Autodesk Inventor part; units mm, degrees
ref_plane "Work Plane1" through (8.5, -35.5, -35.5) normal (0, 0, -1) x (-1, 0, 0)
ref_plane "YZ Plane" through (0, 0, 0) normal (1, 0, 0) x (0, 1, 0)
ref_plane "XZ Plane" through (0, 0, 0) normal (0, 1, 0) x (-1, 0, 0)
ref_plane "Work Plane1" through (8.5, -35.5, -35.5) normal (0, 0, -1) x (-1, 0, 0)
sketch "Sketch1" plane through (8.5, -35.5, -35.5) normal (0, 0, -1) x (-1, 0, 0)
  circle A0 centre (0, 0) radius 3
  circle A1 centre (0, 0) radius 6
  circle A2 centre (-36.75, -21.2176) radius 3
  circle A3 centre (-36.75, -21.2176) radius 6
  circle A4 centre (-36.75, 21.2176) radius 6
  circle A5 centre (-36.75, 21.2176) radius 3
  line L0 (-36.75, -46.2176) -> (28, -46.2176)
  line L1 (28, -46.2176) -> (28, 0)
  line L2 (-36.75, -46.2176) -> (-59, -46.2176)
  line L3 (-59, -46.2176) -> (-59, 34.5)
  line L4 (-59, 34.5) -> (28, 34.5)
  line L5 (34.5, 35.5) -> (-17.5, 35.5)
  line L6 (28, 34.5) -> (28, 0)
  circle A6 centre (-24.5, 0) radius 11
  circle A7 centre (-24.5, 0) radius 15
  point P0 (8.5, 35.5)
  dimension "d3" = 30
extrude "Extrusion1" add sketch "Sketch1" along normal blind 5 contours A1 | A3 | A4 | L2 L3 L4 L6 L1 L0
sketch "Sketch2" plane through (-19.5, -81.7176, -35.5) normal (-1, 0, 0) x (0, 0, 1)
  line L0 (0, 0) -> (0, 80.7176)
  line L1 (0, 80.7176) -> (-5, 80.7176)
  line L2 (-5, 0) -> (-5, 80.7176)
  line L3 (0, 0) -> (-5, 0)
  point P0 (35.5, 81.7176)
extrude "Extrusion2" add sketch "Sketch2" along normal blind 5
sketch "Sketch3" plane through (67.5, -81.7176, -40.5) normal (0, -1, 0) x (1, 0, 0)
  line L0 (0, 5) -> (-92, 5)
  line L1 (-92, 0) -> (-92, 5)
  line L2 (0, 0) -> (-92, 0)
  line L3 (0, 5) -> (0, 0)
  point P0 (-67.5, 40.5)
extrude "Extrusion3" add sketch "Sketch3" along normal blind 5
sketch "Sketch4" plane through (8.5, -35.5, -35.5) normal (0, 0, 1) x (1, 0, 0)
  line L0 (-28, -46.2176) -> (-28, 34.5)
  line L1 (-28, -46.2176) -> (59, -46.2176)
  line L2 (59, -51.2176) -> (-33, -51.2176)
  line L3 (-33, 34.5) -> (-33, -51.2176)
  line L4 (59, 34.5) -> (59, -51.2176)
  line L5 (59, 34.5) -> (-33, 34.5)
  line L6 (-28, -46.2176) -> (-33, -46.2176)
  line L7 (-33, 34.5) -> (-33, -51.2176)
extrude "Extrusion4" add sketch "Sketch4" along normal blind 75 contours L1 L4 L2 L3 L6
sketch "Sketch5" plane through (67.5, -86.7176, -40.5) normal (0, -1, 0) x (1, 0, 0)
  line L0 (-92, 5) -> (-92, 80)
  line L1 (-92, 80) -> (-77.75, 80)
  line L2 (-92, 80) -> (0, 80)
  line L3 (-77.75, 80) -> (-37.75, 80)
  line L4 (-37.75, 80) -> (-37.75, 65)
  line L5 (-37.75, 65) -> (-77.75, 65)
  circle A0 centre (-77.75, 65) radius 4.25
  circle A1 centre (-37.75, 65) radius 4.25
  point P0 (-67.5, 40.5)
  dimension "d14" = 14.25
  dimension "d15" = 40
  dimension "d16" = 15
  dimension "d17" = 8.5
  dimension "d18" = 8.5
extrude "Extrusion5" cut sketch "Sketch5" against normal through all
sketch "Sketch6" plane through (67.5, -1, -35.5) normal (0, 1, 0) x (1, 0, 0)
  line L0 (0, 0) -> (-92, 0)
  line L1 (0, 0) -> (0, 5)
  line L2 (0, 5) -> (-92, 5)
  line L3 (-92, 0) -> (-92, 5)
  point P0 (-67.5, -35.5)
extrude "Extrusion6" add sketch "Sketch6" along normal blind 20
sketch "Sketch7" plane through (67.5, 19, -35.5) normal (0, 1, 0) x (1, 0, 0)
  circle A0 centre (-67.5, -35.5) radius 31
  circle A1 centre (-67.5, -35.5) radius 31
  circle A2 centre (-67.5, -35.5) radius 31
  line L0 (-67.5, -66.5) -> (-67.5, -75)
  line L1 (0, -75) -> (-92, -75)
  line L2 (0, 5) -> (0, -75)
  line L3 (-67.5, -75) -> (0, -75)
  line L4 (0, -75) -> (0, 5)
  line L5 (-65, -20.5) -> (-65, 0)
  line L6 (-65, -4.601) -> (-65, 0)
  line L7 (-92, 5) -> (-92, 0)
  line L8 (-92, 0) -> (0, 0)
  line L9 (0, 0) -> (0, 5)
  line L10 (0, 5) -> (-92, 5)
  point P0 (-65, -4.601)
extrude "Extrusion7" add sketch "Sketch7" along normal blind 20 contours A0 L5 L8 L2 L1 L0 | L8 L7 L10 L2
sketch "Sketch10" plane through (8.5, -35.5, 39.5) normal (0, 0, 1) x (1, 0, 0)
  line L0 (59, -51.2176) -> (59, -46.2176)
  line L1 (59, -46.2176) -> (-33, -46.2176)
  line L2 (-33, -46.2176) -> (-33, -51.2176)
  line L3 (-33, -51.2176) -> (59, -51.2176)
  point P0 (-8.5, 35.5)
extrude "Extrusion10" cut sketch "Sketch10" against normal up to surface (75 mm away)
sketch "Sketch11" plane through (0, 19, 39.5) normal (0, 0, 1) x (1, 0, 0)
  line L0 (0, 0) -> (67.5, 0)
  line L1 (67.5, 0) -> (67.5, 20)
  line L2 (0, 20) -> (67.5, 20)
  line L3 (0, 0) -> (0, 20)
  point P0 (0, -19)
extrude "Extrusion11" add sketch "Sketch11" along normal blind 10
sketch "Sketch12" plane through (67.5, 19, -35.5) normal (0, -1, 0) x (1, 0, 0)
  line L0 (-67.5, 66.5) -> (-67.5, 85)
  line L1 (-67.5, 85) -> (0, 85)
  line L2 (-67.5, 85) -> (0, 85)
  line L3 (0, 85) -> (0, 75)
  line L4 (0, 0) -> (0, 85)
  line L5 (0, 75) -> (-67.5, 75)
  line L6 (-67.5, 75) -> (-67.5, 85)
  point P0 (-67.5, 35.5)
  dimension "d35" = 10
extrude "Extrusion12" add sketch "Sketch12" along normal blind 20
sketch "Sketch13" plane through (0, 19, 49.5) normal (0, 0, 1) x (1, 0, 0)
  line L0 (67.5, 20) -> (67.5, -20)
  line L1 (67.5, 20) -> (0, 20)
  line L2 (0, 20) -> (0, -20)
  line L3 (67.5, -20) -> (0, -20)
  point P0 (0, -19)
extrude "Extrusion13" add sketch "Sketch13" along normal blind 59.488
sketch "Sketch14" plane through (67.5, -1, -35.5) normal (0, -1, 0) x (1, 0, 0)
  line L0 (-53.25, 129.488) -> (-13.25, 129.488)
  circle A0 centre (-53.25, 129.488) radius 4.25
  circle A1 centre (-13.25, 129.488) radius 4.25
  point P0 (-67.5, 35.5)
  point P1 (-67.5, 144.488)
  dimension "d43" = 40
  dimension "d44" = 8.5
  dimension "d45" = 8.5
extrude "Extrusion14" cut sketch "Sketch14" against normal up to surface (40 mm away)
sketch "Sketch15" plane through (67.5, -86.7176, -40.5) normal (1, 0, 0) x (0, 0, -1)
  line L0 (-5, 105.7176) -> (-5, 0)
  line L1 (0, 0) -> (-5, 0)
  line L2 (0, 0) -> (0, 125.7176)
  line L3 (0, 125.7176) -> (-149.488, 125.7176)
  line L4 (-149.488, 85.7176) -> (-149.488, 125.7176)
  line L5 (-80, 85.7176) -> (-149.488, 85.7176)
  line L6 (-80, 105.7176) -> (-80, 85.7176)
  line L7 (-5, 105.7176) -> (-80, 105.7176)
  point P0 (-40.5, 86.7176)
extrude "Extrusion15" add sketch "Sketch15" along normal blind 1
sketch "Sketch16" plane through (0, 19, 31) normal (-1, 0, 0) x (0, 0, 1)
  line L0 (77.988, 20) -> (77.988, -20)
  line L1 (77.988, 0) -> (42.988, 0)
  circle A0 centre (42.988, 0) radius 4.25
  point P0 (-31, -19)
  dimension "d50" = 35
  dimension "d51" = 8.5
extrude "Extrusion16" cut sketch "Sketch16" against normal up to surface (68.5 mm away)
sketch "Sketch17" plane through (67.5, 39, -35.5) normal (0, 1, 0) x (1, 0, 0)
  circle A0 centre (-53.25, -129.488) radius 4.25
  line L0 (-53.25, -129.488) -> (-33.25, -129.488)
  line L1 (-33.25, -129.488) -> (-33.25, -99.488)
  circle A1 centre (-33.25, -99.488) radius 4.25
  point P0 (-67.5, -35.5)
  dimension "d54" = 20
  dimension "d55" = 30
  dimension "d56" = 8.5
extrude "Extrusion17" cut sketch "Sketch17" against normal up to surface (40 mm away) contours A1
sketch "Sketch18" plane through (8.5, -35.5, -35.5) normal (0, 0, 1) x (1, 0, 0)
  line L0 (-6, 54.5) -> (60, 54.5)
  line L1 (-6, 54.5) -> (-6, 74.5)
  line L2 (-33, 74.5) -> (-6, 74.5)
  line L3 (-33, 74.5) -> (-33, -51.2176)
  line L4 (-33, -51.2176) -> (60, -51.2176)
  line L5 (60, 54.5) -> (60, -51.2176)
  circle A0 centre (0, 0) radius 3
  circle A1 centre (36.75, -21.2176) radius 3
  circle A2 centre (36.75, 21.2176) radius 3
  circle A3 centre (24.5, 0) radius 15
  circle A4 centre (36.75, 21.2176) radius 6.5
  circle A5 centre (36.75, -21.2176) radius 6.5
  circle A6 centre (0, 0) radius 3
  circle A7 centre (0, 0) radius 6.5
  point P0 (-8.5, 35.5)
  dimension "d59" = 13
  dimension "d60" = 13
  dimension "d61" = 13
extrude "Extrusion18" add sketch "Sketch18" along normal up to surface (4.601 mm away) contours L0 L5 L4 L3 L2 L1
properties part number "motor_connector_left"
CAD build for the part. Positions are in the model's coordinates, mm. A direction names the side the tool comes from. Give positions to 0.01 mm unless a question says otherwise; leave off trailing zeros. Write each loop counter-clockwise with the first axis right and the second up, starting at its lowest first coordinate (ties: lowest second). Pieces come first, ordered by that corner, then holes. Notation, with made-up numbers: M 51.5,66.25 L 61.5,66.25 A9 cw 61.5,81.25 Z; hole C -8,52 d10. An arc over 180 degrees is marked long. Return JSON: item names as keys, results as strings. Group by question number.
(1) Band-saw the part on B-B (x = 20.5). Give the cut face in (y, z), and give its area (3 significant figures).
(2) Band-saw the part on D-D (y = -5). Give the cut face in (x, z), and give its area (3 significant figures).
(3) Band-saw the part on A-A (x = 54.25). Give the cut face in (y, z).
(4) Flat gauge pins, fed straight in: pin 1 Ø3 at (x, y) = (16.5, -18) entering from +Z; pin 2 Ø4 at (x, y) = (47.5, -56) entering from +Z; pin 3 Ø20.5 at (x, z) = (34, 19) entering from -Y. Where does each tip first touch, or does it go through?
(5) Band-saw the part on C-C (x = 33). Give the cut face in (y, z), and give its area (3 significant figures).
(6) Mould opens along Y. For faces 4 (the face through (21, -25, -40.5)), 5 (the face through (48.247, -14.414, -37.965)), 6 (the face through (21, -86.718, -36)) say: pulls with the +Y half, pulls with the -Y half, needs draft (parallel to the pull), parting line crosses it, or undercut.
(7) Drill centre lines: L1, parallel to X at y = -35, z = -37; L2, parallel to Y at x = 33, z = -37; L3, parallel to X at y = 31.5, z = 64. Where is each one in solid material? Low to high. Write a range as [from, to].
(8) 3-axis set-ups, long thin cutter, end or side, ignore diameter. For faces 1 (the face through (0, 19, 69)), 2 (the face through (41, 19, 4)), 3 (the face through (38.756, -14.568, -33.232)): which of +Z, -Z, +X, -X, +Y, -Y reach the whole face in a straight line?
Entries:
{
 "1": {"outline": "M -86.72,-40.5 L -43.79,-40.5 L -43.79,-30.9 L -86.72,-30.9 Z; M -27.21,-40.5 L 39,-40.5 L 39,-23.25 L 19,-23.25 L 19,-30.9 L -27.21,-30.9 Z; M -1,39.5 L 19,39.5 L 19,23.25 L 39,23.25 L 39,108.99 L -1,108.99 Z; hole C 19,73.99 d8.5", "area": "4,250 mm^2"},
 "2": {"outline": "M -24.5,-40.5 L 68.5,-40.5 L 68.5,-30.9 L -24.5,-30.9 Z", "area": "893 mm^2"},
 "3": {"outline": "M -86.72,-40.5 L 39,-40.5 L 39,89.74 L -1,89.74 L -1,39.5 L 19,39.5 L 19,-30.9 L -86.72,-30.9 Z; M -1,98.24 L 39,98.24 L 39,108.99 L -1,108.99 Z; hole C 19,73.99 d8.5"},
 "4": {"pin 1": "stops at z = -30.9", "pin 2": "stops at z = -35.5", "pin 3": "stops at y = 19"},
 "5": {"outline": "M -86.72,-40.5 L -50.5,-40.5 L -50.5,-30.9 L -86.72,-30.9 Z; M -20.5,-40.5 L 39,-40.5 L 39,59.93 L -1,59.93 L -1,39.5 L 19,39.5 L 19,-30.9 L -20.5,-30.9 Z; M -1,68.05 L 39,68.05 L 39,108.99 L -1,108.99 Z; hole C 19,73.99 d8.5", "area": "4,720 mm^2"},
 "6": {"face 4": "needs draft", "face 5": "undercut", "face 6": "pulls with the -Y half"},
 "7": {"L1": "x = [-24.5, 5.54], [11.46, 18.01], [47.99, 68.5]", "L2": "y = [-86.72, -50.5], [-20.5, 39]", "L3": "x = [0, 30], [38.5, 68.5]"},
 "8": {"face 1": "+Z, -X, +Y, -Y", "face 2": "+X, -X, -Y", "face 3": "+Z"}
}
